from build123d import *

# Parameters (mm, degrees)
SKETCH_R          = 1.75
PAD_DEPTH         = 4
SKETCH001_W       = 4
SKETCH001_H       = 115
PAD001_DEPTH      = 13
SKETCH002_R       = 1.75
SKETCH002_W       = 80
SKETCH002_H       = 9
POCKET_DEPTH      = 10
POCKET_DEPTH_BACK = -5
FILLET_R          = 2


with BuildPart() as part:
    # Sketch → Pad (new body)
    with BuildSketch(Plane.XY):
        Polygon((-17.5, 57.5), (17.5, 57.5), (17.5, 42.5), (5, 42.5), (5, -42.5), (17.5, -42.5), (17.5, -57.5), (-17.5, -57.5), (-17.5, -42.5), (-5, -42.5), (-5, 42.5), (-17.5, 42.5), align=None)
        with Locations((-10, 50)):
            Circle(SKETCH_R, mode=Mode.SUBTRACT)
        with Locations((10, 50)):
            Circle(SKETCH_R, mode=Mode.SUBTRACT)
        with Locations((-10, -50)):
            Circle(SKETCH_R, mode=Mode.SUBTRACT)
        with Locations((10, -50)):
            Circle(SKETCH_R, mode=Mode.SUBTRACT)
    extrude(amount=PAD_DEPTH)

    # Sketch001 → Pad001 (join)
    with BuildSketch(Plane.XY):
        with Locations((-3, 0)):
            Rectangle(SKETCH001_W, SKETCH001_H)
        with Locations((3, 0)):
            Rectangle(SKETCH001_W, SKETCH001_H)
    extrude(amount=PAD001_DEPTH)

    # Sketch002 → Pocket (cut, two sides)
    with BuildSketch(Plane.YZ) as pocket_sk:
        with Locations((45.5, 9)):
            Circle(SKETCH002_R)
        with Locations((-45.5, 9)):
            Circle(SKETCH002_R)
        with Locations((0, 8.5)):
            Rectangle(SKETCH002_W, SKETCH002_H)
    extrude(amount=-POCKET_DEPTH, mode=Mode.SUBTRACT)
    extrude(pocket_sk.sketch, amount=-POCKET_DEPTH_BACK, mode=Mode.SUBTRACT)

    # Fillet
    fillet_edges = [part.edges().sort_by_distance(p)[0] for p in [
        (-3, -40, 13),
        (3, -40, 13),
        (-3, 40, 13),
        (3, 40, 13),
        (-3, 57.5, 13),
        (3, 57.5, 13),
        (17.5, 57.5, 2),
        (17.5, 42.5, 2),
        (3, -57.5, 13),
        (-3, -57.5, 13),
        (17.5, -42.5, 2),
        (17.5, -57.5, 2),
        (-17.5, -42.5, 2),
        (-17.5, -57.5, 2),
        (-17.5, 42.5, 2),
        (-17.5, 57.5, 2),
    ]]
    fillet(fillet_edges, radius=FILLET_R)


solid = part.part
Can you work these out from the model? Positions are in its coordinate system, mm. A direction names the side the tool comes from. Give positions to 0.01 mm unless a question says otherwise; leave off trailing zeros. Loops run counter-clockwise (first coordinate to the right, second up) from the corner with the lowest first, then second, coordinate; pieces in that order, holes last. Notation, with made-up numbers: (50, 8.5) - (76, 8.5) arc R20 cw to (76, 37.5) - close; hole circle Ø4 at (66.5, 19). An arc over 180 degrees is marked (long way). Return JSON: item names as keys, results as strings.
1. For faces 1 (the face through (16.9, -43.07, 2.03)), 2 (the face through (0, 57.5, 3)), 3 (the face through (-3, 40, 7)), which set-ups out of +Z, -Z, +X, -X, +Y, -Y let a thin tool reach every point of the face, with its end or its side?
Output values:
{"face 1": "+Z, -Z, +X", "face 2": "+Z, -Z, +X, -X, +Y", "face 3": "+Z, +X, -X"}
2. I want a section at B-B on y = -50. Please give me the cut outline in (x, z).
Output values:
{"outline": "(-17.5, 0) - (-11.75, 0) - (-11.75, 4) - (-17.5, 4) - close; (-8.25, 0) - (8.25, 0) - (8.25, 4) - (5, 4) - (5, 13) - (1, 13) - (1, 4) - (-1, 4) - (-1, 13) - (-5, 13) - (-5, 4) - (-8.25, 4) - close; (11.75, 0) - (17.5, 0) - (17.5, 4) - (11.75, 4) - close"}
3. We'd pull the mould along Y, two halves only. Please class faces 4 (the face through (-5, -0.8, 3.5)), 5 (the face through (3.03, 40.6, 12.43)), 6 (the face through (3.03, -56.93, 12.4)), 7 (the face through (-3, 49, 13)): +Y half, -Y half, draft (parallel to the pull), parting line (faces both ways), or undercut.
Output values:
{"face 4": "undercut", "face 5": "undercut", "face 6": "-Y half", "face 7": "draft"}
4. I want a section at C-C on x = 10. Please give me the cut outline in (y, z), and give its area (3 significant figures).
Output values:
{"outline": "(-57.5, 0) - (-51.75, 0) - (-51.75, 4) - (-57.5, 4) - close; (-48.25, 0) - (-42.5, 0) - (-42.5, 4) - (-48.25, 4) - close; (42.5, 0) - (48.25, 0) - (48.25, 4) - (42.5, 4) - close; (51.75, 0) - (57.5, 0) - (57.5, 4) - (51.75, 4) - close", "area": "92.0 mm²"}
5. I'm going to push flat-ended pins straight in: pin 1 Ø2.5 at (y, z) = (-49.5, 10) entering from -X; pin 2 Ø8 at (x, y) = (11, 16.5) entering from -Z; pin 3 Ø5.5 at (x, y) = (10, 50) entering from +Z; pin 4 Ø4 at (y, z) = (-45.5, 9) entering from +X. Where does each tip first touch, or does it pass through?
Output values:
{"pin 1": "stops at x = -5", "pin 2": "passes through", "pin 3": "stops at z = 4", "pin 4": "stops at x = 5"}
6. I want a section at D-D on y = -2. Please give me the cut outline in (x, z).
Output values:
{"outline": "(-5, 0) - (5, 0) - (5, 4) - (-5, 4) - close"}
7. I want a section at A-A on z = 9. Give the number of separate pieces and of enclosed holes in the cut face, and give its area (3 significant figures).
Output values:
{"separate pieces": "8", "enclosed holes": "0", "area": "224 mm²"}
8. If I drill on line 1 (Y direction, x = 10, z = 2.85); line 2 (Y direction, x = -13.5, z = 1); line 3 (Y direction, x = -1.5, z = 8.5), over which ranges is the centre line in solid material (lowest first)?
Output values:
{"line 1": "y = -57.5 to -51.75, -48.25 to -42.5, 42.5 to 48.25, 51.75 to 57.5", "line 2": "y = -57.5 to -42.5, 42.5 to 57.5", "line 3": "y = -57.5 to -47.18, -43.82 to -40, 40 to 43.82, 47.18 to 57.5"}
